Verification items for the finished model (mm, model axes). Face numbers are marked on the shaded views. A direction names the side the tool comes from. Coordinates: 2 decimals unless noted, no trailing zeros. Order: outer loops, then holes, each group sorted by start corner. A loop starts at its lowest first (then second) coordinate and runs counter-clockwise, first axis right, second up.
Q1. Set-up check for the marked faces 1 and 2: record each of +Z, -Z, +X, -X, +Y, -Y from which the full face is reachable in a straight line by a thin tool's end or side.
Q2. Depth check by flat-ended pin: P1, Ø1, axis at x = -26, z = 5, coming from the +Y side; P2, Ø1, axis at x = 14.5, y = 3, coming from the +Z side; P3, Ø6, axis at y = -6.5, z = -10, coming from the +X side. Enter the tip coordinate at first touch or a pass-through.
Q3. Thickness scan on line 1 (X direction, y = 2, z = -1); line 2 (Z direction, x = 7, y = -9.5); line 3 (X direction, y = -5, z = -16). Record the ranges inside material, lowest first.
Q4. Cross-section at A-A, the plane z = 3. Record the boundary of the cut face in (x, y).
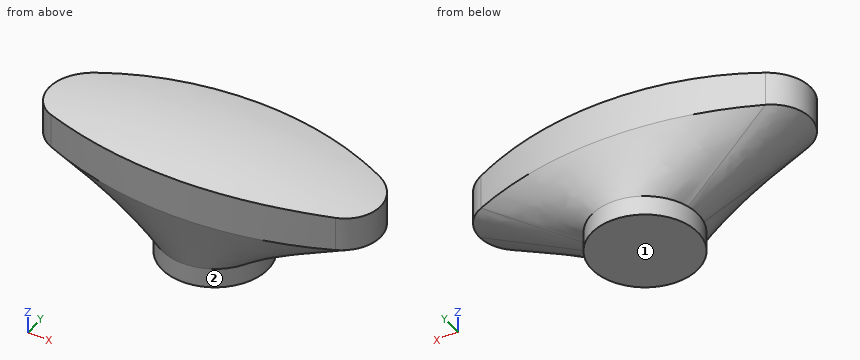
from build123d import *

# Parameters (mm, degrees)
SKETCH001_R  = 13.5
PAD_DEPTH    = 12
PAD001_DEPTH = 5


with BuildPart() as part:
    # Sketch → AdditiveLoft section 0
    with BuildSketch(Plane.XY):
        with BuildLine():
            ThreePointArc((-36.562505, 9.137617), (-42.5, 6e-06), (-36.562516, -9.137612))
            ThreePointArc((-36.562516, -9.137612), (-9e-06, -16.899042), (36.5625, -9.13762))
            ThreePointArc((36.5625, -9.13762), (42.5, 0), (36.5625, 9.13762))
            ThreePointArc((36.5625, 9.13762), (-3e-06, 16.899042), (-36.562505, 9.137617))
        make_face()
    # Sketch001 → AdditiveLoft section 1
    with BuildSketch(Plane.XY.offset(-15)):
        Circle(SKETCH001_R)
    loft()

    # Sketch → Pad (new body)
    with BuildSketch(Plane.XY):
        with BuildLine():
            ThreePointArc((-36.562505, 9.137617), (-42.5, 6e-06), (-36.562516, -9.137612))
            ThreePointArc((-36.562516, -9.137612), (-9e-06, -16.899042), (36.5625, -9.13762))
            ThreePointArc((36.5625, -9.13762), (42.5, 0), (36.5625, 9.13762))
            ThreePointArc((36.5625, 9.13762), (-3e-06, 16.899042), (-36.562505, 9.137617))
        make_face()
    extrude(amount=PAD_DEPTH)

    # Sketch001 → Pad001 (join)
    with BuildSketch(Plane.XY.offset(-15)):
        Circle(SKETCH001_R)
    extrude(amount=-PAD001_DEPTH)

    # SubtractivePipe: sweep along a path in Sketch002
    with BuildLine(Plane.XZ) as subtractivepipe_path:
        ThreePointArc((54.893133, 5.916665), (0.078349, 12), (-54.736434, 5.916665))
    # Sketch003 → SubtractivePipe (sweep, cut)
    with BuildSketch(Plane.YZ):
        with BuildLine():
            ThreePointArc((33.346504, 4.178945), (1.160914, 11.991015), (-31.251067, 5.178962))
            Line((-31.251067, 5.178962), (-31.251067, 34.885342))
            Line((-31.251067, 34.885342), (33.346504, 34.885342))
            Line((33.346504, 34.885342), (33.346504, 4.178945))
        make_face()
    sweep(path=subtractivepipe_path.line, mode=Mode.SUBTRACT)


solid = part.part
Check values:
1. face 1: -Z, +X, -X, +Y, -Y
1. face 2: -Z
2. P1: stops at y = 13.21
2. P2: stops at z = 11.56
2. P3: stops at x = 26.4
3. line 1: x = -40.36 to 40.36
3. line 2: z = -20 to 11.3
3. line 3: x = -12.54 to 12.54
4. outline: (-36.56, -9.14) arc R90 ccw to (36.56, -9.14) arc R10 ccw to (36.56, 9.14) arc R90 ccw to (-36.56, 9.14) arc R10 ccw to start
